Verification items for the finished model (mm, model axes). Face numbers are marked on the shaded views. Round coordinates to 2 decimals unless told otherwise and drop trailing zeros. Write each loop counter-clockwise with the first axis right and the second up, starting at its lowest first coordinate (ties: lowest second). Pieces come first, ordered by that corner, then holes. Notation, with made-up numbers: M 0.25,32.5 L 31.25,32.5 A12 cw 31.25,46.5 Z; hole C -33.75,-39.75 d10. An arc over 180 degrees is marked long. One line per item, written item: value. Start each with the question number.
Item 1: Section check A-A, the plane x = 0. Record the cut outline in (y, z), then the cut area to 3 significant figures.
Item 2: Draft check along Z on the marked faces 1 and 2. Enter one of: +Z half, -Z half, draft (parallel to the pull), parting line (faces both ways), or undercut.
Item 3: Thickness scan on probe 1 along Z at (x, y) = (0, 0.35); probe 2 along X at (y, z) = (0.5, 0); probe 3 along X at (y, z) = (-2.2, -84). Record the ranges inside material, lowest first. Write a range as from..to.
Item 4: Section check C-C, the plane z = -11. Record the cut outline in (x, y), then the cut area to 3 significant figures.
Item 5: Section check D-D, the plane x = 5.5. Record the cut outline in (y, z), then the cut area to 3 significant figures.
Item 6: Gauge pin test, flat ends, axial feed: pin 1 (2 mm diameter, centred on x = -0.5, z = -0.5, fed in from -Y); pin 2 (3 mm diameter, centred on x = 3, z = -80.5, fed in from -Y); pin 3 (1 mm diameter, centred on x = -9.5, z = -4, fed in from -Y). Record the tip position at first contact, or that the pin passes through.
Item 7: Section check B-B, the plane z = -66.5. Record the cut outline in (x, y).
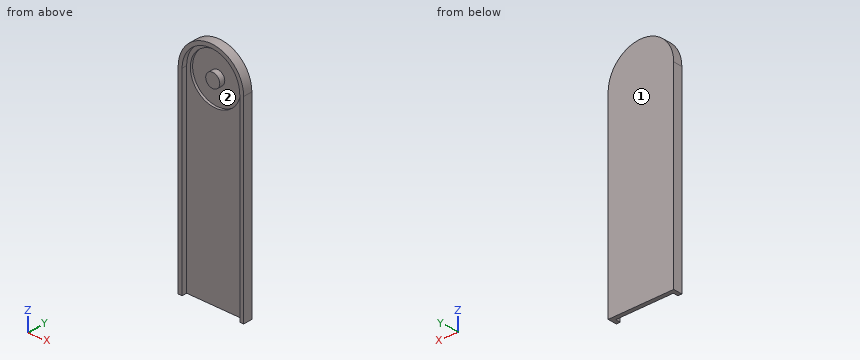
Autodesk Fusion 360 part; units mm, degrees
sketch "Sketch1" plane through (0, 0, 0) normal (0, 1, 0) x (1, 0, 0)
  line L0 (-16.3, 0) -> (16.3, 0)
  line L1 (16.3, 0) -> (16.3, 97.5)
  line L2 (16.3, 97.5) -> (-16.3, 97.5)
  line L3 (-16.3, 97.5) -> (-16.3, 0)
  line L4 (0, 102.6744) -> (0, -20) construction
  arc A0 (-16.3, 0) -> (16.3, 0) centre (0, 0) ccw
  line L5 (-14.35, 97.5) -> (-14.35, 0)
  arc A1 (-14.35, 0) -> (14.35, 0) centre (0, 0) ccw
  line L6 (14.35, 0) -> (14.35, 97.5)
  dimension "d1" = 32.6
  dimension "d2" = 97.5
  dimension "d3" = 1.95
extrude "Extrude1" add sketch "Sketch1" along normal blind 2
extrude "Extrude2" add sketch "Sketch1" against normal blind 2.5 contours L0 L2 L3 L5 | L0 A0 A1 | L0 L1 L2 L6
sketch "Sketch2" plane through (0, 0, 7.15) normal (0, 1, 0) x (1, 0, 0)
  circle A0 centre (0, 7.15) radius 3.5
  circle A1 centre (0, 7.15) radius 4.1
  circle A2 centre (0, 7.15) radius 4.7
  circle A3 centre (0, 7.15) radius 5.3
  circle A4 centre (0, 7.15) radius 5.9
  circle A5 centre (0, 7.15) radius 6.5
  circle A6 centre (0, 7.15) radius 7.1
  circle A7 centre (0, 7.15) radius 7.7
  circle A8 centre (0, 7.15) radius 8.3
  line L0 (27.1083, -9.4638) -> (28.3083, -9.4638)
  line L1 (28.3083, -9.4638) -> (28.3083, -7.488)
  line L2 (28.3083, -7.488) -> (27.1083, -7.488)
  line L3 (27.1083, -7.488) -> (27.1083, -9.4638)
  circle A9 centre (0, 7.15) radius 8.9
  circle A10 centre (0, 7.15) radius 9.5
  circle A11 centre (0, 7.15) radius 10.1
  circle A12 centre (0, 7.15) radius 10.7
  circle A13 centre (0, 7.15) radius 11.3
  circle A14 centre (0, 7.15) radius 11.9
  circle A15 centre (0, 7.15) radius 12.5
  dimension "d18" = 7
  dimension "d19" = 8.2
  dimension "d20" = 1.2
  dimension "d21" = 9.4
  dimension "d22" = 10.6
  dimension "d23" = 11.8
  dimension "d24" = 13
  dimension "d25" = 14.2
  dimension "d26" = 15.4
  dimension "d27" = 16.6
  dimension "d28" = 17.8
  dimension "d29" = 19
  dimension "d30" = 20.2
  dimension "d31" = 21.4
  dimension "d32" = 22.6
  dimension "d33" = 23.8
  dimension "d34" = 25
extrude "Extrude4" cut sketch "Sketch2" along normal blind 1.25 contours A1 | A2 | A3 | A4 | A5 | A6 | A7 | A8 | A9 | A10 | A11 | A12 | A13 | A14 | A15
extrude "Extrude5" add 1 faces at (0.555, 0, 0.9381) along direction (0, -1, 0) blind 1.5
equation "d1 = 33 mm - 0.4 mm"
equation "d2 = 114 mm - ( 33 / 2 ) * 1 mm"
equation "d19 = d18 + d20"
equation "d21 = d19 + d20"
equation "d22 = d21 + d20"
equation "d23 = d22 + d20"
equation "d24 = d23 + d20"
equation "d25 = d24 + d20"
equation "d26 = d25 + d20"
equation "d27 = d26 + d20"
equation "d28 = d27 + d20"
equation "d29 = d28 + d20"
equation "d30 = d29 + d20"
equation "d31 = d30 + d20"
equation "d32 = d31 + d20"
equation "d33 = d32 + d20"
equation "d34 = d33 + d20"
Response values:
1. outline: M -2.5,14.35 L 0,14.35 L 0,12.5 L 1.25,12.5 L 1.25,3.5 L -1.5,3.5 L -1.5,-3.5 L 1.25,-3.5 L 1.25,-12.5 L 0,-12.5 L 0,-97.5 L 2,-97.5 L 2,16.3 L -2.5,16.3 Z
1. area: 220 mm2
2. face 1: draft
2. face 2: undercut
3. probe 1: z = -97.5..-12.5, -3.5..3.5, 12.5..16.3
3. probe 2: x = -16.3..-12.5, -3.5..3.5, 12.5..16.3
3. probe 3: x = -16.3..-14.35, 14.35..16.3
4. outline: M -16.3,-2.5 L -14.35,-2.5 L -14.35,0 L -5.94,0 L -5.94,1.25 L 5.94,1.25 L 5.94,0 L 14.35,0 L 14.35,-2.5 L 16.3,-2.5 L 16.3,2 L -16.3,2 Z
4. area: 60.1 mm2
5. outline: M -2.5,13.25 L 0,13.25 L 0,11.22 L 1.25,11.22 L 1.25,-11.22 L 0,-11.22 L 0,-97.5 L 2,-97.5 L 2,15.34 L -2.5,15.34 Z
5. area: 203 mm2
6. pin 1: stops at y = -1.5
6. pin 2: stops at y = 0
6. pin 3: stops at y = 1.25
7. outline: M -16.3,-2.5 L -14.35,-2.5 L -14.35,0 L 14.35,0 L 14.35,-2.5 L 16.3,-2.5 L 16.3,2 L -16.3,2 Z
